Job drawing, mm, ordinate dimensions from the low corner. One solid piece. A direction names the side the tool comes from. Give positions to 0.01 mm unless a question says otherwise; leave off trailing zeros. Write each loop counter-clockwise with the first axis right and the second up, starting at its lowest first coordinate (ties: lowest second). Pieces come first, ordered by that corner, then holes. Notation, with made-up numbers: M 57.25,10.5 L 71.25,10.5 A27 ccw 71.25,38.5 Z; hole C 62,17.5 d5. An arc over 180 degrees is marked long. Use CSV: the item, a comma, the result in double quotes. Start each with the question number.
Item 1: Cut at C-C (z = 45). List the corners of the cut face in (x, y), then the cut area to 3 significant figures.
Item 2: Cut at A-A (x = 15). List the corners of the cut face in (y, z).
Item 3: Drill centre lines: line 1 (Z direction, x = 125, y = 77); line 2 (Y direction, x = 37, z = 21.5); line 3 (Y direction, x = 50.5, z = 5.5). Where is each one in solid material? Low to high. Write a range as [from, to].
Item 4: Mould opens along Y. For the marked faces 6, 7 and 8 say: released by +Y, released by -Y, zero draft, split by the parting line, or undercut.
Item 5: Pin check, flat tips, straight feed: pin 1 (15 mm diameter, centred on x = 132, z = 52, fed in from -Y); pin 2 (2 mm diameter, centred on y = 32, z = 47.5, fed in from -X); pin 3 (9 mm diameter, centred on x = 120.5, y = 33, fed in from +Z). Stop position of each tip, or through.
Item 6: Cut at B-B (y = 73.5). List the corners of the cut face in (x, z).
Item 7: Cut at D-D (y = 45). List the corners of the cut face in (x, z).
Item 8: Which spindle directions (+Z, -Z, +X, -X, +Y, -Y) get a long thin tool onto all of the face, cutting with end or side? Do the marked faces 1, 2, 3, 4 and 5. Say none if no direction does.
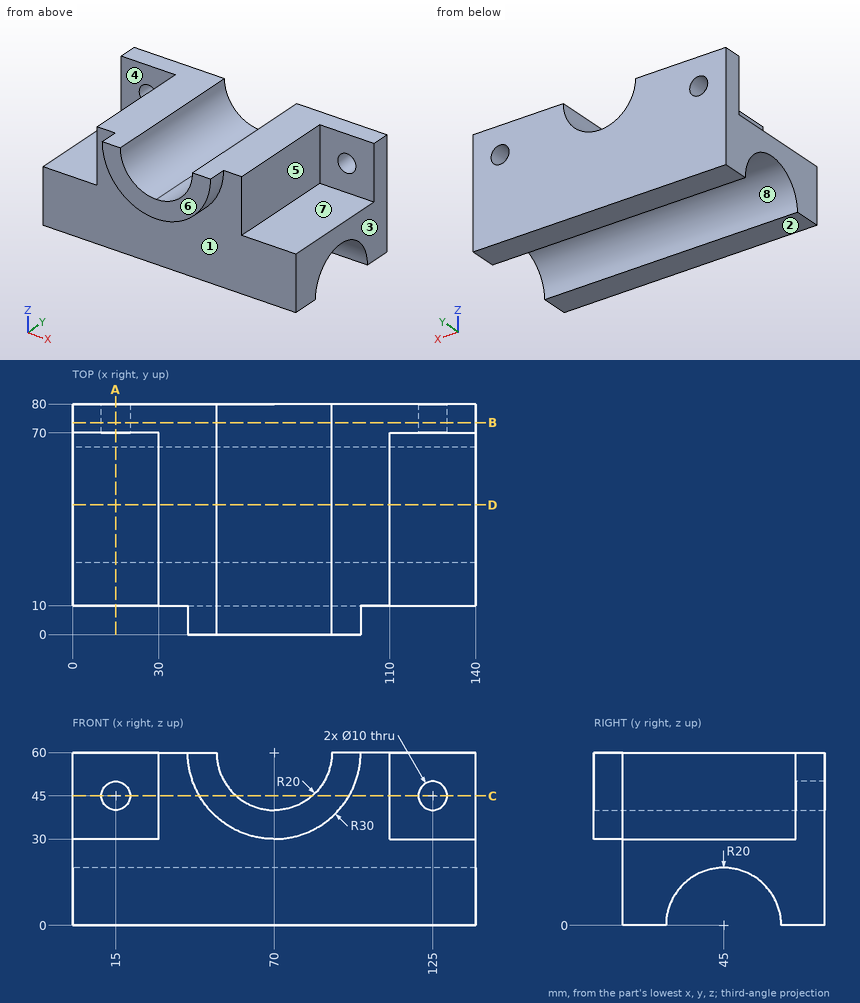
Worked answers:
1,outline,"M 0,70 L 10,70 L 10,80 L 0,80 Z; M 20,70 L 30,70 L 30,10 L 44.02,10 L 44.02,0 L 56.77,0 L 56.77,80 L 20,80 Z; M 83.23,0 L 95.98,0 L 95.98,10 L 110,10 L 110,70 L 120,70 L 120,80 L 83.23,80 Z; M 130,70 L 140,70 L 140,80 L 130,80 Z"
1,area,"4,400 mm^2"
2,outline,"M 10,0 L 25,0 A20 cw 65,0 L 80,0 L 80,40 L 70,40 L 70,30 L 10,30 Z; M 70,50 L 80,50 L 80,60 L 70,60 Z"
3,line 1,"z = [0, 40], [50, 60]"
3,line 2,"y = [10, 80]"
3,line 3,"y = [10, 25.77], [64.23, 80]"
4,face 6,"released by -Y"
4,face 7,"zero draft"
4,face 8,"undercut"
5,pin 1,"stops at y = 70"
5,pin 2,"stops at x = 30"
5,pin 3,"stops at z = 30"
6,outline,"M 0,0 L 140,0 L 140,60 L 90,60 A20 cw 70,40 A20 cw 50,60 L 0,60 Z; hole C 15,45 d10; hole C 125,45 d10"
7,outline,"M 0,20 L 140,20 L 140,30 L 110,30 L 110,60 L 90,60 A20 cw 70,40 A20 cw 50,60 L 30,60 L 30,30 L 0,30 Z"
8,face 1,"-Z, -Y"
8,face 2,"-Z, +X, -X, +Y, -Y"
8,face 3,"+Z, -Z, +X, +Y, -Y"
8,face 4,"+Z, -X, -Y"
8,face 5,"+Z, +X, -Y"
